from build123d import *


with BuildPart() as f1:
    # F0 (on Front) → F1 (revolve)
    with BuildSketch(Plane.XZ):
        with BuildLine():
            Line((-61.5, 0), (-1, 0))
            Line((-1, 0), (-1, 0.5))
            Line((-1, 0.5), (-61.5, 0.5))
            Line((-61.5, 0.5), (-61.5, 164.293947))
            ThreePointArc((-61.5, 164.293947), (-62.436346, 164.737428), (-63.438581, 165))
            Line((-63.438581, 165), (-65.25, 165))
            ThreePointArc((-65.25, 165), (-67.379659, 164.175331), (-69, 162.565976))
            Line((-69, 162.565976), (-67.530356, 162.565976))
            ThreePointArc((-67.530356, 162.565976), (-65.25873, 164.183882), (-62.5, 163.774847))
            Line((-62.5, 163.774847), (-62.5, 162.919664))
            Line((-62.5, 162.919664), (-62.5, 0.5))
            ThreePointArc((-62.5, 0.5), (-62.353553, 0.146447), (-62, 0))
            Line((-62, 0), (-61.5, 0))
        make_face()
    revolve(axis=Axis((-1, 0, 17.714524), (0, 0, 1)))


solid = f1.part
CAD build for the part. Positions are in the model's coordinates, mm. A direction names the side the tool comes from. Give positions to 0.01 mm unless a question says otherwise; leave off trailing zeros. Loops run counter-clockwise (first coordinate to the right, second up) from the corner with the lowest first, then second, coordinate; pieces in that order, holes last. Notation, with made-up numbers: M 52,46 L 69,46 A23 ccw 69,68 Z; hole C 26,13 d1. An arc over 180 degrees is marked long. Answer in a Markdown table with one row per item. Add a question column.
Item 1: Band-saw the part on A-A on x = -1. Give the cut face in (y, z).
Item 2: Mould opens along Y. For faces 4 (the face through (-54, -34, 165)), 5 (the face through (-2, -1, 0.5)), 6 (the face through (-29.38, 54.56, 80.99)) say: +Y half, -Y half, draft (parallel to the pull), parting line (faces both ways), or undercut.
Item 3: Tool access for faces 1 (the face through (-46, 50, 162.566)), 2 (the face through (12.12, 59.06, 83.54)), 3 (the face through (0, -1, 0)): list every direction of +Z, -Z, +X, -X, +Y, -Y with a clear straight run to the whole face (end or side of a thin tool).
Item 4: Band-saw the part on B-B on z = 54.5. Give the cut face in (x, y), then the cut area to 3 significant figures.
Item 5: Probe probe 1 along Y at (x, z) = (-1, 127.5); probe 2 along X at (y, z) = (0, 75); probe 3 along Z at (x, y) = (41.5, -41.5). List the from-to ranges inside material, lowest first.
Item 6: Band-saw the part on C-C on y = 0. Give the cut face in (x, z).
Item 7: Drop flat-ended pins along their axis: P1, Ø10, axis at y = -1, z = 102, coming from the -X side; P2, Ø12, axis at x = -4, y = 37.5, coming from the +Z side; P3, Ø1, axis at x = 1.5, z = 64.5, coming from the -Y side. Give the stop position or say it passes through.
Reply:
| question | item | result |
|---|---|---|
| 1 | outline | M -68,162.57 L -66.53,162.57 A3.73 cw -61.5,163.77 L -61.5,0.5 A0.5 ccw -61,0 L 61,0 A0.5 ccw 61.5,0.5 L 61.5,163.77 A3.73 cw 66.53,162.57 L 68,162.57 A5.58 ccw 64.25,165 L 62.44,165 A5.58 ccw 60.5,164.29 L 60.5,0.5 L -60.5,0.5 L -60.5,164.29 A5.58 ccw -62.44,165 L -64.25,165 A5.58 ccw Z |
| 2 | face 4 | draft |
| 2 | face 5 | undercut |
| 2 | face 6 | parting line |
| 3 | face 1 | -Z |
| 3 | face 2 | +Z |
| 3 | face 3 | -Z, +X, -X, +Y, -Y |
| 4 | outline | C -1,0 d123; hole C -1,0 d121 |
| 4 | area | 383 mm^2 |
| 5 | probe 1 | y = -61.5 to -60.5, 60.5 to 61.5 |
| 5 | probe 2 | x = -62.5 to -61.5, 59.5 to 60.5 |
| 5 | probe 3 | z = 0 to 0.5 |
| 6 | outline | M -69,162.57 L -67.53,162.57 A3.73 cw -62.5,163.77 L -62.5,0.5 A0.5 ccw -62,0 L 60,0 A0.5 ccw 60.5,0.5 L 60.5,163.77 A3.73 cw 65.53,162.57 L 67,162.57 A5.58 ccw 63.25,165 L 61.44,165 A5.58 ccw 59.5,164.29 L 59.5,0.5 L -61.5,0.5 L -61.5,164.29 A5.58 ccw -63.44,165 L -65.25,165 A5.58 ccw Z |
| 7 | P1 | stops at x = -62.5 |
| 7 | P2 | stops at z = 0.5 |
| 7 | P3 | stops at y = -61.47 |
